Geometry: final body of the model. Coordinates: model frame, mm. A direction names the side the tool comes from. Round coordinates to 2 decimals unless told otherwise and drop trailing zeros. Order: outer loops, then holes, each group sorted by start corner. A loop starts at its lowest first (then second) coordinate and runs counter-clockwise, first axis right, second up. Notation, with made-up numbers: M 44,0 L 73,0 A16 ccw 73,12 Z; hole C -21.5,-25.5 d11. An arc over 180 degrees is marked long. Put each result on its own line as item: value. Start each with the question number.
1) Section B-B, the plane z = -140. Return loops of the section in (x, y), then the cut area to 3 significant figures.
2) Draft query along X for faces 4 (the flat face through (0, 4, -76)), 5 (the flat face through (2, -2, -66)), 6 (the flat face through (10.5, 2, -139)), 7 (the flat face through (-18, 2, -139)). Return one class per face: pulls with the +X half, pulls with the -X half, needs draft (parallel to the pull), parting line crosses it, or undercut.
3) Section D-D, the plane z = -76.5. Return loops of the section in (x, y).
4) First-contact query: P1, Ø1.7, axis at x = 5, z = -163.91, coming from the +Y side; P2, Ø1.5, axis at x = -1.5, z = -81, coming from the -Y side; P3, Ø3, axis at x = 11.5, y = 1.5, coming from the +Z side; P4, Ø1.2, axis at y = 2, z = 11, coming from the -X side. Flat tips, straight axial feed; report the tip coordinate or a pass-through.
5) Material intervals for probe 1 along X at (y, z) = (1.4, -115.28); probe 2 along Z at (x, y) = (-6.5, 1.25) (3 decimals); probe 3 along Z at (x, y) = (-5.5, 2.25) (3 decimals), sorted ascending. Write a range as [from, to].
6) Section C-C, the plane x = 13. Return loops of the section in (y, z) (3 decimals), then the cut area to 3 significant figures.
7) Access query for faces 1 (the cylindrical face through (0, 2, 18)), 2 (the cylindrical face through (3.51, 1.97, -3.56)), 3 (the cylindrical face through (-16.04, 2.03, -15.21)). Directions: +Z, -Z, +X, -X, +Y, -Y. A direction counts if a zero-diameter tool reaches every point of the face in a straight line with its end or side. Return the directions, or none.
8) Section A-A, the plane y = 2.5. Count the separate pieces of the cut face and the enclosed holes in it, then the cut area to 3 significant figures.
from build123d import *

# Parameters (mm, degrees)
SKETCH_1_R          = 1.45
SKETCH_1_W          = 21
SKETCH_1_H          = 41
EXTRUDE_1_DEPTH     = 4
CUT_EXTRUDE_1_DEPTH = 170.103308735
EXTRUDE_2_DEPTH     = 2


with BuildPart() as part:
    # 스케치1 → 보스-돌출1 (new body)
    with BuildSketch(Plane(origin=(0, 0, 0), x_dir=(1, 0, 0), z_dir=(0, 1, 0))):
        with BuildLine():
            Line((18, 0), (18, 168.095))
            Line((18, 168.095), (-18, 168.095))
            Line((-18, 168.095), (-18, 0))
            ThreePointArc((-18, 0), (0, -18), (18, 0))
        make_face()
        with BuildLine():
            ThreePointArc((-15, -1.2), (-16.2, 0), (-15, 1.2))
            Line((-15, 1.2), (-4.85386444, 1.2))
            ThreePointArc((-4.85386444, 1.2), (-3.535533906, 3.535533906), (-1.2, 4.85386444))
            Line((-1.2, 4.85386444), (-1.2, 15))
            ThreePointArc((-1.2, 15), (0, 16.2), (1.2, 15))
            Line((1.2, 15), (1.2, 4.85386444))
            ThreePointArc((1.2, 4.85386444), (3.535533906, 3.535533906), (4.85386444, 1.2))
            Line((4.85386444, 1.2), (15, 1.2))
            ThreePointArc((15, 1.2), (16.2, 0), (15, -1.2))
            Line((15, -1.2), (4.85386444, -1.2))
            ThreePointArc((4.85386444, -1.2), (3.535533906, -3.535533906), (1.2, -4.85386444))
            Line((1.2, -4.85386444), (1.2, -15))
            ThreePointArc((1.2, -15), (0, -16.2), (-1.2, -15))
            Line((-1.2, -15), (-1.2, -4.85386444))
            ThreePointArc((-1.2, -4.85386444), (-3.535533906, -3.535533906), (-4.85386444, -1.2))
            Line((-4.85386444, -1.2), (-15, -1.2))
        make_face(mode=Mode.SUBTRACT)
        with Locations(Location((-5, 115.28, 0), (0, 0, 270))):
            Circle(SKETCH_1_R, mode=Mode.SUBTRACT)
        with Locations(Location((-5, 163.91, 0), (0, 0, 270))):
            Circle(SKETCH_1_R, mode=Mode.SUBTRACT)
        with Locations(Location((5, 115.28, 0), (0, 0, 270))):
            Circle(SKETCH_1_R, mode=Mode.SUBTRACT)
        with Locations((0, 139.595)):
            Rectangle(SKETCH_1_W, SKETCH_1_H, mode=Mode.SUBTRACT)
        with Locations(Location((5, 163.91, 0), (0, 0, 270))):
            Circle(SKETCH_1_R, mode=Mode.SUBTRACT)
    extrude(amount=EXTRUDE_1_DEPTH)

    # 스케치2 → 컷-돌출1 (cut, through all)
    with BuildSketch(Plane(origin=(0, 4, 0), x_dir=(1, 0, 0), z_dir=(0, 1, 0))):
        with BuildLine():
            Line((-18, 110), (-10.5, 102.5))
            Line((-10.5, 102.5), (-10.5, 29.047375097))
            ThreePointArc((-10.5, 29.047375097), (-16.094750193, 15), (-18, 0))
            Line((-18, 0), (-18, 110))
        make_face()
    cut_extrude_1 = extrude(amount=-CUT_EXTRUDE_1_DEPTH, mode=Mode.SUBTRACT)

    # 대칭 복사1: 컷-돌출1 across plane
    add(cut_extrude_1.mirror(Plane(origin=(0, 0, 0), x_dir=(0, 0, 1), z_dir=(1, 0, 0))), mode=Mode.SUBTRACT)

    # 스케치3 → 보스-돌출2 (add, symmetric)
    with BuildSketch(Plane(origin=(0, 0, 0), x_dir=(0, 0, -1), z_dir=(1, 0, 0))):
        with BuildLine():
            Line((25, 0), (105, 0))
            ThreePointArc((105, 0), (65, -5.431677052), (25, 0))
        make_face()
    extrude(amount=EXTRUDE_2_DEPTH, both=True)


solid = part.part
Result sheet:
1. outline: M -18,0 L -10.5,0 L -10.5,4 L -18,4 Z; M 10.5,0 L 18,0 L 18,4 L 10.5,4 Z
1. area: 60.0 mm2
2. face 4: needs draft
2. face 5: pulls with the +X half
2. face 6: undercut
2. face 7: pulls with the -X half
3. outline: M -10.5,0 L -2,0 L -2,-4.99 L 2,-4.99 L 2,0 L 10.5,0 L 10.5,4 L -10.5,4 Z
4. P1: passes through
4. P2: stops at y = -4.65
4. P3: stops at z = 14.97
4. P4: stops at x = -14.69
5. probe 1: x = [-18, -6.45], [-3.55, 3.55], [6.45, 18]
5. probe 2: z = [-168.095, -160.095], [-119.095, -1.2], [1.2, 16.785]
5. probe 3: z = [-168.095, -165.271], [-162.549, -160.095], [-119.095, -116.641], [-113.919, -1.2], [1.2, 17.139]
6. outline: M 0,-168.095 L 4,-168.095 L 4,-105 L 0,-105 Z; M 0,-23.979 L 4,-23.979 L 4,-1.2 L 0,-1.2 Z; M 0,1.2 L 4,1.2 L 4,12.45 L 0,12.45 Z
6. area: 388 mm2
7. face 1: +Z, +Y, -Y
7. face 2: +Y, -Y
7. face 3: -X, +Y, -Y
8. separate pieces: 1
8. enclosed holes: 6
8. area: 4,190 mm2
